```python
from build123d import *

# Parameters (mm, degrees)
BOSS_EXTRUDE4_DEPTH = 10
SKETCH5_R           = 1.6210620194390177
BOSS_EXTRUDE8_DEPTH = 10
CIRPATTERN4_COUNT   = 5
SKETCH6_R           = 9.321133181207394
BOSS_EXTRUDE9_DEPTH = 10
CUT_EXTRUDE1_DEPTH  = 10
FILLET1_R           = 10


with BuildPart() as part:
    # Sketch3 → Boss-Extrude4 (new body)
    with BuildSketch(Plane(origin=(0, 0, 0), x_dir=(1, 0, 0), z_dir=(0, 1, 0))):
        with BuildLine():
            ThreePointArc((-2.568584889231257, 0), (-15.859987880186992, 40.28882096120527), (3.4054490784254314, 78.086882111293))
            ThreePointArc((3.4054490784254314, 78.086882111293), (4.310285634950187, 78.05431633363062), (5.144295315107662, 77.70187119279029))
            ThreePointArc((5.144295315107662, 77.70187119279029), (-9.176823691930053, 42.2861657946719), (-2.568584889231257, 4.660405757344381))
            ThreePointArc((-2.568584889231257, 4.660405757344381), (-2.7066052458532077, 2.3302028786721882), (-2.568584889231257, 0))
        make_face()
    extrude(amount=BOSS_EXTRUDE4_DEPTH)


with BuildPart() as body_2:
    # Sketch5 → Boss-Extrude8 (new body)
    with BuildSketch(Plane(origin=(0, 0, 0), x_dir=(1, 0, 0), z_dir=(0, 1, 0))):
        with Locations(Location((0, 0, 0), (0, 0, 270))):
            Circle(SKETCH5_R)
    extrude(amount=BOSS_EXTRUDE8_DEPTH)


with BuildPart() as cirpattern4_1:
    # CirPattern4: pattern copy
    add(part.part.rotate(Axis((-3.4e-16, 0, -5.8e-16), (0, 1, 0)), 1 * 360 / CIRPATTERN4_COUNT))


with BuildPart() as cirpattern4_2:
    # CirPattern4: pattern copy
    add(part.part.rotate(Axis((-3.4e-16, 0, -5.8e-16), (0, 1, 0)), 2 * 360 / CIRPATTERN4_COUNT))


with BuildPart() as cirpattern4_3:
    # CirPattern4: pattern copy
    add(part.part.rotate(Axis((-3.4e-16, 0, -5.8e-16), (0, 1, 0)), 3 * 360 / CIRPATTERN4_COUNT))


with BuildPart() as cirpattern4_4:
    # CirPattern4: pattern copy
    add(part.part.rotate(Axis((-3.4e-16, 0, -5.8e-16), (0, 1, 0)), 4 * 360 / CIRPATTERN4_COUNT))


with BuildPart() as part_1:
    add(part.part)

    add(body_2.part)  # Boss-Extrude9 merges body 2

    add(cirpattern4_1.part)  # Boss-Extrude9 merges CirPattern4_1

    add(cirpattern4_2.part)  # Boss-Extrude9 merges CirPattern4_2

    add(cirpattern4_3.part)  # Boss-Extrude9 merges CirPattern4_3

    add(cirpattern4_4.part)  # Boss-Extrude9 merges CirPattern4_4
    # Sketch6 → Boss-Extrude9 (add)
    with BuildSketch(Plane(origin=(0, 10, 0), x_dir=(1, 0, 0), z_dir=(0, 1, 0))):
        Circle(SKETCH6_R)
    extrude(amount=-BOSS_EXTRUDE9_DEPTH)

    # Sketch7 → Cut-Extrude1 (cut)
    with BuildSketch(Plane(origin=(0, 10, 0), x_dir=(1, 0, 0), z_dir=(0, 1, 0))):
        with BuildLine():
            Line((1.1925707526180573, 2.78), (-1.1925707526180573, 2.78))
            ThreePointArc((-1.1925707526180578, 2.78), (-1.6647970556993392, -2.5256832270367577), (3.025, -7.4e-16))
            ThreePointArc((3.025, 0), (2.5256832270367577, 1.6647970556993388), (1.1925707526180576, 2.78))
        make_face()
    extrude(amount=-CUT_EXTRUDE1_DEPTH, mode=Mode.SUBTRACT)

    # Fillet1
    # the kernel refuses this fillet: 10 mm, written as the material it adds along each edge
    with BuildSketch(Plane(origin=(9.294704214468556, 10, 0.7014252257691618), x_dir=(0.9166930954116449, 0, 0.399592002953784), z_dir=(0, -1, 0))) as fillet1_piece_1:
        with BuildLine():
            CenterArc((5.437298438361188, -9.98977111966082), FILLET1_R, 92.59172373372462, 44.87729573930281)
            ThreePointArc((-1.9318208534579913, -3.2298834828033556), (-0.8012017224871335, -1.713455421939968), (0, 0))
            ThreePointArc((0, 0), (2.4925557778833074, -0.0563838885471548), (4.985111555766614, 2e-17))
        make_face()
    extrude(amount=10)
    with BuildSketch(Plane(origin=(6.60253368503394, 10, -6.579519186065028), x_dir=(0.46308073985482195, 0, 0.8863160995804548), z_dir=(0, -1, 0))) as fillet1_piece_2:
        with BuildLine():
            CenterArc((8.524117810925986, -9.546886996079968), FILLET1_R, 107.3138862206167, 66.77214806671216)
            ThreePointArc((-1.4226595103454045, -8.516537093842318), (-0.8440182810230222, -4.236103365094945), (0, 0))
            ThreePointArc((0, 0), (2.774027598326007, -0.42235266556755513), (5.548055196652016, 2e-17))
        make_face()
    extrude(amount=10)
    with BuildSketch(Plane(origin=(-4.2171994813875955, 10, -8.31256592851991), x_dir=(-0.3267162956046077, 0, -0.9451224588308135), z_dir=(0, -1, 0))) as fillet1_piece_3:
        with BuildLine():
            CenterArc((8.011945209416133, 9.980599667944867), FILLET1_R, 206.79739354469726, 66.7721480667119)
            ThreePointArc((-0.9141180755940358, 5.47223031395517), (-0.04047863659748981, 2.805703542850818), (0, 0))
            ThreePointArc((0, 0), (4.317272407237243, -0.13452709830263468), (8.634544814474475, -3.1e-16))
        make_face()
    extrude(amount=10)
    with BuildSketch(Plane(origin=(3.539316591620801, 10, -8.623036695160394), x_dir=(-0.9827141698360341, 0, -0.18512930725164625), z_dir=(0, -1, 0))) as fillet1_piece_4:
        with BuildLine():
            CenterArc((5.782329586263011, 9.794100565483701), FILLET1_R, 213.47572744282695, 44.87729573930915)
            ThreePointArc((-2.5588660900526423, 4.278263848410483), (-1.2310439268876425, 2.1680738683956533), (0, 0))
            ThreePointArc((0, 0), (1.881759756341037, 0.19192160510617215), (3.7635195126820715, -5e-17))
        make_face()
    extrude(amount=10)
    with BuildSketch(Plane(origin=(-9.208906301869895, 10, 1.4420709085153902), x_dir=(-0.9998257608489958, 0, 0.018666760370418967), z_dir=(0, -1, 0))) as fillet1_piece_5:
        with BuildLine():
            CenterArc((8.011945209416153, 9.980599667944865), FILLET1_R, 206.79739354469731, 66.7721480667119)
            ThreePointArc((-0.9141180755940117, 5.472230313955157), (-0.04047863659747148, 2.8057035428508104), (0, 0))
            ThreePointArc((0, 0), (4.317272407237252, -0.13452709830265147), (8.634544814474507, -2e-17))
        make_face()
    extrude(amount=10)
    with BuildSketch(Plane(origin=(-7.1072862639004715, 10, -6.030754989615849), x_dir=(-0.47974381311129005, 0, 0.8774086127805217), z_dir=(0, -1, 0))) as fillet1_piece_6:
        with BuildLine():
            CenterArc((5.782329586263038, 9.794100565483692), FILLET1_R, 213.47572744282687, 44.877295739309034)
            ThreePointArc((-2.5588660900526223, 4.278263848410486), (-1.2310439268876405, 2.168073868395652), (0, 0))
            ThreePointArc((0, 0), (1.8817597563410384, 0.19192160510617853), (3.763519512682072, -7e-17))
        make_face()
    extrude(amount=10)
    with BuildSketch(Plane(origin=(-7.931861070486542, 10, 4.895825133754791), x_dir=(-0.9764945790844407, 0, 0.21554196115536567), z_dir=(0, -1, 0))) as fillet1_piece_7:
        with BuildLine():
            CenterArc((5.43729843836118, -9.989771119660821), FILLET1_R, 92.59172373372459, 44.877295739302724)
            ThreePointArc((-1.9318208534579884, -3.2298834828033454), (-0.801201722487141, -1.7134554219399574), (0, 0))
            ThreePointArc((0, 0), (2.492555777883305, -0.05638388854715234), (4.985111555766614, 5e-17))
        make_face()
    extrude(amount=10)
    with BuildSketch(Plane(origin=(-1.4742176123811461, 10, 9.203814764169852), x_dir=(-0.8956037205130516, 0, -0.44485275744135816), z_dir=(0, -1, 0))) as fillet1_piece_8:
        with BuildLine():
            CenterArc((8.524117810925947, -9.546886996079973), FILLET1_R, 107.31388622061658, 66.77214806671205)
            ThreePointArc((-1.422659510345439, -8.516537093842285), (-0.8440182810230522, -4.236103365094935), (0, 0))
            ThreePointArc((0, 0), (2.774027598325997, -0.42235266556755147), (5.548055196651995, 2.3e-16))
        make_face()
    extrude(amount=10)
    with BuildSketch(Plane(origin=(2.2051265282976815, 10, 9.056541325252308), x_dir=(-0.0967608331602571, 0, 0.9953076615630632), z_dir=(0, -1, 0))) as fillet1_piece_9:
        with BuildLine():
            CenterArc((5.437298438361169, -9.989771119660823), FILLET1_R, 92.59172373372452, 44.87729573930274)
            ThreePointArc((-1.9318208534579957, -3.229883482803339), (-0.8012017224871391, -1.7134554219399516), (0, 0))
            ThreePointArc((0, 0), (2.4925557778833074, -0.05638388854715363), (4.985111555766614, 3e-17))
        make_face()
    extrude(amount=10)
    with BuildSketch(Plane(origin=(8.297789710604665, 10, 4.2461994418996625), x_dir=(-0.6998368836204316, 0, 0.7143026923681881), z_dir=(0, -1, 0))) as fillet1_piece_10:
        with BuildLine():
            CenterArc((8.52411781092599, -9.546886996079968), FILLET1_R, 107.3138862206167, 66.77214806671219)
            ThreePointArc((-1.4226595103454007, -8.516537093842324), (-0.8440182810230218, -4.236103365094961), (0, 0))
            ThreePointArc((0, 0), (2.774027598326008, -0.4223526655675579), (5.548055196652019, 1.7e-16))
        make_face()
    extrude(amount=10)


solid = part_1.part
```
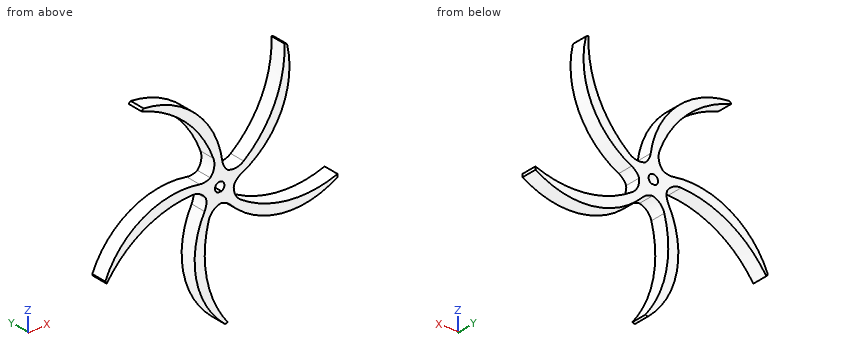
Geometry check sheet. Reference: the model listing, model coordinates, mm. Round coordinates to 2 decimals unless told otherwise and drop trailing zeros. Order: outer loops, then holes, each group sorted by start corner. A loop starts at its lowest first (then second) coordinate and runs counter-clockwise, first axis right, second up. Notation, with made-up numbers: (28, -7) - (64, -7) arc R20 ccw to (64, 2) - close; hole circle Ø4 at (-38.75, 29.25). An arc over 180 degrees is marked (long way). Use a Markdown table: item, result. Add a question column.
1) Gauge pin test, flat ends, axial feed: P1, Ø6, axis at y = 5.5, z = 31, coming from the -X side; P2, Ø1.5, axis at x = 48.5, y = 6.5, coming from the -Z side; P3, Ø6, axis at x = 23, y = 3, coming from the -Z side. Record the tip position at first contact, or that the pin passes through.
2) Thickness scan on line 1 along X through (y, z) = (3, 38.5); line 2 along Z through (x, y) = (-37, 8.5); line 3 along Z through (x, y) = (21, 3). Record the ranges inside material, lowest first.
3) Section check A-A (x = 31). Record the cut outline in (y, z), then the cut area to 3 significant figures.
4) Section check B-B (z = 39). Record the cut outline in (x, y).
5) Section check D-D (x = 61). Record the cut outline in (y, z), then the cut area to 3 significant figures.
Established:
| question | item | result |
|---|---|---|
| 1 | P1 | x = -12.89 |
| 1 | P2 | z = -29.07 |
| 1 | P3 | z = -25.17 |
| 2 | line 1 | -16.46 to -8.17, 36.91 to 42.97 |
| 2 | line 2 | -1.97 to 4.77, 54.73 to 59.01 |
| 2 | line 3 | -22.88 to -16.1, 6.89 to 14.18 |
| 3 | outline | (0, -26.89) - (10, -26.89) - (10, -20.12) - (0, -20.12) - close; (0, 15.81) - (10, 15.81) - (10, 26.69) - (0, 26.69) - close |
| 3 | area | 176 mm2 |
| 4 | outline | (-16.89, 0) - (-8.54, 0) - (-8.54, 10) - (-16.89, 10) - close; (37.1, 0) - (43.1, 0) - (43.1, 10) - (37.1, 10) - close |
| 5 | outline | (0, -27.12) - (10, -27.12) - (10, -22.69) - (0, -22.69) - close |
| 5 | area | 44.3 mm2 |
